Autodesk Inventor part; units mm, degrees
ref_plane "YZ Plane" through (0, 0, 0) normal (1, 0, 0) x (0, 1, 0)
ref_plane "XZ Plane" through (0, 0, 0) normal (0, 1, 0) x (-1, 0, 0)
ref_plane "XY Plane" through (0, 0, 0) normal (0, 0, 1) x (1, 0, 0)
sketch "Sketch1" plane through (0, 0, 0) normal (0, 0, 1) x (1, 0, 0)
  line L0 (0, 0) -> (0, 73)
  line L1 (0, 73) -> (25.5, 73)
  line L2 (25.5, 73) -> (25.5, 63)
  line L3 (25.5, 63) -> (12.5, 63)
  line L4 (12.5, 63) -> (12.5, 44)
  line L5 (12.5, 44) -> (5, 44)
  line L6 (5, 44) -> (5, 0)
  line L7 (5, 0) -> (0, 0)
  dimension "d0" = 25.5
  dimension "d1" = 10
  dimension "d2" = 19
  dimension "d3" = 12.5
  dimension "d4" = 44
  dimension "d5" = 5
revolve "Revolution1" add sketch "Sketch1" angle 360 about axis through (0, 0, 0) along (0, 1, 0)
properties part number "Knob"
CAD build for the part. Positions are in the model's coordinates, mm. A direction names the side the tool comes from. Round coordinates to 2 decimals unless told otherwise and drop trailing zeros. Write each loop counter-clockwise with the first axis right and the second up, starting at its lowest first coordinate (ties: lowest second). Pieces come first, ordered by that corner, then holes. Notation, with made-up numbers: (17.25, 25) -> (29.25, 25) arc R22 cw to (29.25, 38) -> close; hole circle Ø6 at (26, 22.5). An arc over 180 degrees is marked (long way). Answer in a Markdown table with one row per item. Add a question column.
Item 1: Which spindle directions (+Z, -Z, +X, -X, +Y, -Y) get a long thin tool onto all of the face, cutting with end or side? Do faces 1 (the face through (-5.5, 67.9, -24.9)), 2 (the face through (-1.08, 21.69, -4.88)). Say none if no direction does.
Item 2: Drop flat-ended pins along their axis: pin 1 Ø5 at (y, z) = (35, 9) entering from -X; pin 2 Ø4 at (x, z) = (13.5, -2.5) entering from -Y; pin 3 Ø12.5 at (x, z) = (-2, 5.5) entering from -Y; pin 4 Ø1 at (x, y) = (-7.5, 55) entering from -Z. Give the stop position or say it passes through.
Item 3: Saw through at C-C, the plane y = 49. Write the cut outline in (x, z), then the cut area to 3 significant figures.
Item 4: Saw through at B-B, the plane x = 0. Write the cut outline in (y, z).
Item 5: Saw through at D-D, the plane x = 9.5. Write the cut outline in (y, z), then the cut area to 3 significant figures.
Item 6: Drill centre lines: line 1 (Y direction, x = -3, z = -8); line 2 (Y direction, x = 17, z = -4.5); line 3 (X direction, y = 52.5, z = 0.5). Where is each one in solid material? Low to high. Write a range as from..to.
Item 7: Saw through at A-A, the plane z = 0. Write the cut outline in (x, y).
Findings below:
| question | item | result |
|---|---|---|
| 1 | face 1 | +Y, -Y |
| 1 | face 2 | -Y |
| 2 | pin 1 | passes through |
| 2 | pin 2 | stops at y = 44 |
| 2 | pin 3 | stops at y = 0 |
| 2 | pin 4 | stops at z = -10.36 |
| 3 | outline | circle Ø25 at (0, 0) |
| 3 | area | 491 mm^2 |
| 4 | outline | (0, -5) -> (44, -5) -> (44, -12.5) -> (63, -12.5) -> (63, -25.5) -> (73, -25.5) -> (73, 25.5) -> (63, 25.5) -> (63, 12.5) -> (44, 12.5) -> (44, 5) -> (0, 5) -> close |
| 5 | outline | (44, -8.12) -> (63, -8.12) -> (63, -23.66) -> (73, -23.66) -> (73, 23.66) -> (63, 23.66) -> (63, 8.12) -> (44, 8.12) -> close |
| 5 | area | 782 mm^2 |
| 6 | line 1 | y = 44..73 |
| 6 | line 2 | y = 63..73 |
| 6 | line 3 | x = -12.49..12.49 |
| 7 | outline | (-25.5, 63) -> (-12.5, 63) -> (-12.5, 44) -> (-5, 44) -> (-5, 0) -> (5, 0) -> (5, 44) -> (12.5, 44) -> (12.5, 63) -> (25.5, 63) -> (25.5, 73) -> (-25.5, 73) -> close |
